The listing builds one solid part. Answer for the finished solid, in the listing's coordinates (mm). Face numbers are marked on the shaded views. A direction names the side the tool comes from. Coordinates: 2 decimals unless noted, no trailing zeros. Write each loop counter-clockwise with the first axis right and the second up, starting at its lowest first coordinate (ties: lowest second). Pieces come first, ordered by that corner, then holes.
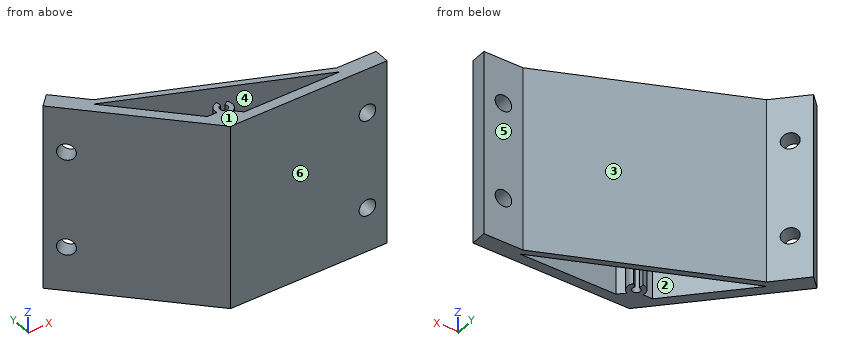
from build123d import *

# Parameters (mm, degrees)
EXTRUDE_1_DEPTH         = 48
HOLE_WIZARD_8_5_8_5_1_D = 8.5


with BuildPart() as part:
    # 草图1 → 凸台-拉伸1 (new, symmetric)
    with BuildSketch(Plane.XY):
        Polygon((6936.119122288, -1232.086390659), (6992.687664783, -1288.654933154), (7072.687664783, -1288.654933154), (7072.687664783, -1280.654933154), (7052.687664783, -1280.654933154), (6955.918112162, -1240.571672033), (6941.775976538, -1226.429536409), align=None)
        with BuildLine():
            Line((7009.090927681, -1283.654933154), (7003.090927681, -1283.654933154))
            Line((7003.090927681, -1283.654933154), (6999.760549745, -1280.324555218))
            ThreePointArc((6999.760549745, -1280.324555218), (7002.213755914, -1277.239517812), (7001.296666197, -1273.406161221))
            Line((7001.296666197, -1273.406161221), (6999.365595427, -1274.993916141))
            ThreePointArc((6999.365595427, -1274.993916141), (6997.055371947, -1278.111879141), (6997.626530039, -1274.273571671))
            Line((6997.626530039, -1274.273571671), (6997.383769074, -1271.785386165))
            ThreePointArc((6997.383769074, -1271.785386165), (6994.101203016, -1273.731324494), (6993.49338103, -1277.49861375))
            Line((6993.49338103, -1277.49861375), (6988.602413191, -1277.49861375))
            Line((6988.602413191, -1277.49861375), (6954.21874867, -1243.114949228))
            Line((6954.21874867, -1243.114949228), (7052.090927681, -1283.654933154))
            Line((7052.090927681, -1283.654933154), (7029.403393536, -1283.654933154))
            Line((7029.403393536, -1283.654933154), (7009.090927681, -1283.654933154))
        make_face(mode=Mode.SUBTRACT)
    extrude(amount=EXTRUDE_1_DEPTH, both=True)

    # Ø8.5 (8.5) 直径孔1 (through all)
    with Locations(Plane(origin=(2852.016365815, 2852.016365815, 0), x_dir=(0.7071067811865628, -0.7071067811865324, 0), z_dir=(-0.7071067811865324, -0.7071067811865628, 0))):
        with Locations((5785.79350833, -25), (5785.79350833, 25)):
            hole_wizard_8_5_8_5_1 = Hole(HOLE_WIZARD_8_5_8_5_1_D / 2)

    # 镜向1: Ø8.5 (8.5) 直径孔1 across plane
    add(hole_wizard_8_5_8_5_1.mirror(Plane(origin=(6424.240586557, -2661.0075789, 0), x_dir=(0, 0, 1), z_dir=(-0.9238795325112645, 0.3826834323651437, 0))), mode=Mode.SUBTRACT)


solid = part.part
Q1. Given pin 1 (2 mm diameter, centred on y = -1269, z = -30, fed in from +X); pin 2 (2 mm diameter, centred on y = -1234, z = 6.5, fed in from +X); pin 3 (22 mm diameter, centred on x = 7062, z = 24, fed in from +Y), each flat-ended and moving along its own axis, determine where each tip first touches the part or whether it passes through.
Answers below:
pin 1: stops at x = 7026.96
pin 2: stops at x = 6950.35
pin 3: stops at y = -1279.96
Q2. The part is cut by section C-C, the plane y = -1263. Write down the section's boundary in (x, z), then the cut area to 3 significant figures.
Answers below:
outline: (6967.03, -48) - (6974.1, -48) - (6974.1, 48) - (6967.03, 48) - close; (7002.23, -48) - (7010.06, -48) - (7010.06, 48) - (7002.23, 48) - close
area: 1,430 mm2
Q3. Determine the mould class of the marked faces 1, 2 and 3 for opening direction X: released by +X, released by -X, zero draft, split by the parting line, or undercut.
Answers below:
face 1: zero draft
face 2: undercut
face 3: released by +X
Q4. The part is cut by section A-A, the plane z = -25. Write down the section's boundary in (x, y), then the cut area to 3 significant figures.
Answers below:
outline: (6936.12, -1232.09) - (6940.18, -1236.15) - (6945.84, -1230.5) - (6941.78, -1226.43) - close; (6946.2, -1242.16) - (6992.69, -1288.65) - (7058.44, -1288.65) - (7058.44, -1280.65) - (7052.69, -1280.65) - (6955.92, -1240.57) - (6951.85, -1236.51) - close; (7066.94, -1288.65) - (7072.69, -1288.65) - (7072.69, -1280.65) - (7066.94, -1280.65) - close; hole (6954.22, -1243.11) - (6988.6, -1277.5) - (6993.49, -1277.5) arc R4.5 cw to (6997.38, -1271.79) - (6997.63, -1274.27) arc R2 ccw (long way) to (6999.37, -1274.99) - (7001.3, -1273.41) arc R4.5 cw to (6999.76, -1280.32) - (7003.09, -1283.65) - (7052.09, -1283.65) - close
area: 1,170 mm2
Q5. The part is cut by section D-D, the plane z = -0.5. Write down the section's boundary in (x, y), then the cut area to 3 significant figures.
Answers below:
outline: (6936.12, -1232.09) - (6992.69, -1288.65) - (7072.69, -1288.65) - (7072.69, -1280.65) - (7052.69, -1280.65) - (6955.92, -1240.57) - (6941.78, -1226.43) - close; hole (6954.22, -1243.11) - (6988.6, -1277.5) - (6993.49, -1277.5) arc R4.5 cw to (6997.38, -1271.79) - (6997.63, -1274.27) arc R2 ccw (long way) to (6999.37, -1274.99) - (7001.3, -1273.41) arc R4.5 cw to (6999.76, -1280.32) - (7003.09, -1283.65) - (7052.09, -1283.65) - close
area: 1,310 mm2
Q6. Find the intervals of material crossed by probe 1 along X at (y, z) = (-1282.5, -25); probe 2 along X at (y, z) = (-1274.5, -38.5); probe 3 along X at (y, z) = (-1276, -11), in increasing order.
Answers below:
probe 1: x = 6986.53 to 7001.94, 7049.3 to 7058.44, 7066.94 to 7072.69
probe 2: x = 6978.53 to 6985.6, 6993.68 to 6996.88, 6999.97 to 7001.96, 7029.99 to 7037.83
probe 3: x = 6980.03 to 6987.1, 6993.33 to 6995.84, 6999.8 to 7002.31, 7033.61 to 7041.45
Q7. Which of the six approach directions +Z, -Z, +X, -X, +Y, -Y give full straight-line access (tool end or side, diameter ignored) to the marked faces 4, 5 and 6?
Answers below:
face 4: +Z, -Z
face 5: +Z, -Z, +X, +Y
face 6: +Z, -Z, +X, -X, -Y
Q8. The part is cut by section B-B, the plane x = 7008. Write down the section's boundary in (y, z), then the cut area to 3 significant figures.
Answers below:
outline: (-1288.65, -48) - (-1283.65, -48) - (-1283.65, 48) - (-1288.65, 48) - close; (-1265.39, -48) - (-1262.14, -48) - (-1262.14, 48) - (-1265.39, 48) - close
area: 792 mm2
